Part model, mm, in its own coordinate system. A direction names the side the tool comes from. Give positions to 0.01 mm unless a question says otherwise; leave off trailing zeros. Loops run counter-clockwise (first coordinate to the right, second up) from the corner with the lowest first, then second, coordinate; pieces in that order, holes last. Notation, with made-up numbers: M 35,-1.5 L 58,-1.5 A28 ccw 58,33.5 Z; hole C -10.75,3.5 d5. An arc over 180 degrees is marked long. Answer in a Markdown table with one row per item.
from build123d import *

# Parameters (mm, degrees)
SKETCH1_W                       = 8
SKETCH1_H                       = 90
SKETCH1_R                       = 3.1
BOSS_EXTRUDE1_DEPTH             = 4
FILLET1_R                       = 4
BOSS_EXTRUDE2_START             = -4
SKETCH2_R                       = 7.5
SKETCH2_R_2                     = 3.1
BOSS_EXTRUDE2_DEPTH             = 4
SKETCH3_W                       = 2
SKETCH3_H                       = 78.65571123
CUT_EXTRUDE2_DEPTH              = 49.254533466
SKETCH4_W                       = 1
SKETCH4_H                       = 78.65571123
SKETCH5_W                       = 13.19082965
SKETCH5_H                       = 5
BOSS_EXTRUDE5_DEPTH             = 10
BOSS_EXTRUDE5_DIRECTION_2_REACH = 50.255


with BuildPart() as part:
    # Sketch1 → Boss-Extrude1 (new body)
    with BuildSketch(Plane(origin=(0, 0, 0), x_dir=(1, 0, 0), z_dir=(0, 1, 0))):
        Rectangle(SKETCH1_W, SKETCH1_H)
        with Locations(Location((0, -40, 0), (0, 0, 270))):
            Circle(SKETCH1_R, mode=Mode.SUBTRACT)
    extrude(amount=BOSS_EXTRUDE1_DEPTH)

    # Fillet1
    fillet1_edges = [part.edges().sort_by_distance(p)[0] for p in [
        (-4, 2, 45),
        (4, 2, 45),
    ]]
    fillet(fillet1_edges, radius=FILLET1_R - 0.0001)  # a hair under: the kernel refuses the full size

    # Sketch2 → Boss-Extrude2 (add)
    with BuildSketch(Plane(origin=(0, 4, 0), x_dir=(1, 0, 0), z_dir=(0, 1, 0)).offset(BOSS_EXTRUDE2_START)):
        with Locations((0, -40)):
            Circle(SKETCH2_R)
        with Locations(Location((0, -40, 0), (0, 0, 270))):
            Circle(SKETCH2_R_2, mode=Mode.SUBTRACT)
    extrude(amount=BOSS_EXTRUDE2_DEPTH)

    # Sketch3 → Cut-Extrude2 (cut, through all)
    with BuildSketch(Plane(origin=(0, 4, 0), x_dir=(1, 0, 0), z_dir=(0, 1, 0))):
        with Locations((3, 5.672144385)):
            Rectangle(SKETCH3_W, SKETCH3_H)
        with Locations((-3, 5.672144385)):
            Rectangle(SKETCH3_W, SKETCH3_H)
    extrude(amount=-CUT_EXTRUDE2_DEPTH, mode=Mode.SUBTRACT)

    # Sketch4 → Revolve1 (revolve)
    with BuildSketch(Plane.XZ):
        with Locations((-0.5, -5.672144385)):
            Rectangle(SKETCH4_W, SKETCH4_H)
    revolve(axis=Axis((0, 0, 40), (0, 0, -1)))

    # Sketch5 → Boss-Extrude5 (add)
    with BuildSketch(Plane.XZ):
        with Locations((1.5, -42.5)):
            Rectangle(SKETCH5_W, SKETCH5_H)
    extrude(amount=BOSS_EXTRUDE5_DEPTH)

    # Boss-Extrude5 direction 2: up to this face of the body (flat: up to its plane)
    boss_extrude5_direction_2_end = Plane(part.part.faces().sort_by_distance((0, 4, 8.504231921))[0])
    # Sketch5 → Boss-Extrude5 direction 2 (add, up to the picked face)
    with BuildSketch(Plane.XZ, mode=Mode.PRIVATE) as boss_extrude5_direction_2_sk1:
        with Locations((1.5, -42.5)):
            Rectangle(SKETCH5_W, SKETCH5_H)
    boss_extrude5_direction_2_tool1 = split(extrude(boss_extrude5_direction_2_sk1.sketch, amount=-BOSS_EXTRUDE5_DIRECTION_2_REACH, mode=Mode.PRIVATE), bisect_by=boss_extrude5_direction_2_end, keep=Keep.BOTH, mode=Mode.PRIVATE)
    add(boss_extrude5_direction_2_tool1.solids().sort_by(Axis((1.5, 0, -42.5), (0, 1, 0)))[0])


solid = part.part
(1) Pull direction Z, two halves, no side cores. Call faces 4 (the face through (3, 2, 33.656)), 5 (the face through (1, -10, -42)), 6 (the face through (1, -3, -45)): +Z half, -Z half, draft (parallel to the pull), parting line (faces both ways), or undercut.
Recorded:
| item | result |
|---|---|
| face 4 | undercut |
| face 5 | draft |
| face 6 | -Z half |
(2) Pin check, flat tips, straight feed: pin 1 Ø2.5 at (y, z) = (0, -43) entering from -X; pin 2 Ø5 at (x, z) = (0, 40) entering from +Y; pin 3 Ø4.5 at (y, z) = (3, -18) entering from +X; pin 4 Ø1.2 at (y, z) = (2.5, -13.5) entering from -X. Stop position of each tip, or through.
Recorded:
| item | result |
|---|---|
| pin 1 | stops at x = -5.1 |
| pin 2 | passes through |
| pin 3 | stops at x = 2 |
| pin 4 | stops at x = -2 |
(3) Drill centre lines: line 1 along X through (y, z) = (0.9, 40); line 2 along Y through (x, z) = (-5.5, 41); line 3 along X through (y, z) = (3.25, 32). Where is each one in solid material? Low to high.
Recorded:
| item | result |
|---|---|
| line 1 | x = -7.5 to -3.1, 3.1 to 7.5 |
| line 2 | y = 0 to 4 |
| line 3 | x = -2 to 2 |
(4) Saw through at C-C (x = 0). Write the cut outline in (y, z), plus the area to 3 significant figures.
Recorded:
| item | result |
|---|---|
| outline | M -10,-45 L 4,-45 L 4,36.9 L 0,36.9 L 0,33.66 L -1,33.66 L -1,-40 L -10,-40 Z; M 0,43.1 L 4,43.1 L 4,47.5 L 0,47.5 Z |
| area | 469 mm^2 |
(5) Saw through at A-A (x = 6). Write the cut outline in (y, z), plus the area to 3 significant figures.
Recorded:
| item | result |
|---|---|
| outline | M -10,-45 L 4,-45 L 4,-40 L -10,-40 Z; M 0,35.5 L 4,35.5 L 4,44.5 L 0,44.5 Z |
| area | 106 mm^2 |
(6) Saw through at D-D (y = -4.5). Write the cut outline in (x, z).
Recorded:
| item | result |
|---|---|
| outline | M -5.1,-45 L 8.1,-45 L 8.1,-40 L -5.1,-40 Z |
(7) Which spindle directions (+Z, -Z, +X, -X, +Y, -Y) get a long thin tool onto all of the face, cutting with end or side? Do faces 1 (the face through (0, -1, -3)), 2 (the face through (-3, 2, 33.656)), 3 (the face through (2, 2, -3)). Say none if no direction does.
Recorded:
| item | result |
|---|---|
| face 1 | +Z, -Y |
| face 2 | -X, +Y, -Y |
| face 3 | +X, +Y, -Y |
(8) Saw through at B-B (z = 40). Write the cut outline in (x, y).
Recorded:
| item | result |
|---|---|
| outline | M -7.5,0 L -3.1,0 L -3.1,4 L -7.5,4 Z; M 3.1,0 L 7.5,0 L 7.5,4 L 3.1,4 Z |
